Geometry check sheet. Reference: the model listing, model coordinates, mm. A direction names the side the tool comes from. Round coordinates to 2 decimals unless told otherwise and drop trailing zeros. Order: outer loops, then holes, each group sorted by start corner. A loop starts at its lowest first (then second) coordinate and runs counter-clockwise, first axis right, second up.
(1) Cross-section at A-A on x = 16. Enter the section's corners in (y, z), and give its area (3 significant figures).
(2) Cross-section at D-D on x = -41. Enter the section's corners in (y, z).
(3) Cross-section at C-C on y = 22.5. Enter the section's corners in (x, z), and give its area (3 significant figures).
(4) Set-up check for faces 5 (the face through (-1, 27.5, 1)), 6 (the face through (12.75, 14, 1)): record each of +Z, -Z, +X, -X, +Y, -Y from which the full face is reachable in a straight line by a thin tool's end or side.
(5) Cross-section at B-B on y = 0. Enter the section's corners in (x, z), and give its area (3 significant figures).
(6) Thickness scan on L1, parallel to X at y = 12, z = 2.9; L2, parallel to Y at x = -4.5, z = 2.55; L3, parallel to Y at x = 41, z = 2.3. Record the ranges inside material, lowest first.
(7) Draft check along X on faces 1 (the face through (-35.391, 16.796, 1.479)), 2 (the face through (1, 21, 1)), 3 (the face through (46, 0, 1)), 4 (the face through (-1, 0, 3)). Enter one of: pulls with the +X half, pulls with the -X half, needs draft (parallel to the pull), parting line crosses it, or undercut.
from build123d import *

# Parameters (mm, degrees)
SKETCH1_W           = 92
SKETCH1_H           = 55
SKETCH1_R           = 2
SKETCH1_R_2         = 1.5
BOSS_EXTRUDE1_DEPTH = 3


with BuildPart() as part:
    # Sketch1 → Boss-Extrude1 (new body)
    with BuildSketch(Plane.XY):
        Rectangle(SKETCH1_W, SKETCH1_H)
        with Locations((-34, 0)):
            Circle(SKETCH1_R, mode=Mode.SUBTRACT)
        with Locations((-14, 0)):
            Circle(SKETCH1_R, mode=Mode.SUBTRACT)
        with Locations((16, 0)):
            Circle(SKETCH1_R, mode=Mode.SUBTRACT)
        with Locations((-41, 22.5)):
            Circle(SKETCH1_R_2, mode=Mode.SUBTRACT)
        with Locations((41, 22.5)):
            Circle(SKETCH1_R_2, mode=Mode.SUBTRACT)
        with Locations((41, -22.5)):
            Circle(SKETCH1_R_2, mode=Mode.SUBTRACT)
        with Locations((-41, -22.5)):
            Circle(SKETCH1_R_2, mode=Mode.SUBTRACT)
        with BuildLine():
            Line((12.75, -21), (12.75, -6.199798384))
            ThreePointArc((12.75, -6.199798384), (11.050252532, -4.949747468), (9.800201616, -3.25))
            Line((9.800201616, -3.25), (-7.800201616, -3.25))
            ThreePointArc((-7.800201616, -3.25), (-9.050252532, -4.949747468), (-10.75, -6.199798384))
            Line((-10.75, -6.199798384), (-10.75, -21))
            Line((-10.75, -21), (12.75, -21))
        make_face(mode=Mode.SUBTRACT)
        with BuildLine():
            Line((-39.5, 4.330127019), (-39.5, 14.641883177))
            ThreePointArc((-39.5, 14.641883177), (-35.343145751, 16.843145751), (-33.141883177, 21))
            Line((-33.141883177, 21), (-17.25, 21))
            Line((-17.25, 21), (-17.25, 6.199798384))
            ThreePointArc((-17.25, 6.199798384), (-18.949747468, 4.949747468), (-20.199798384, 3.25))
            Line((-20.199798384, 3.25), (-27.800201616, 3.25))
            ThreePointArc((-27.800201616, 3.25), (-33.356495502, 6.970358812), (-39.5, 4.330127019))
        make_face(mode=Mode.SUBTRACT)
        with BuildLine():
            Line((-27.800201616, -3.25), (-20.199798384, -3.25))
            ThreePointArc((-20.199798384, -3.25), (-18.949747468, -4.949747468), (-17.25, -6.199798384))
            Line((-17.25, -6.199798384), (-17.25, -21))
            Line((-17.25, -21), (-33.141883177, -21))
            ThreePointArc((-33.141883177, -21), (-35.343145751, -16.843145751), (-39.5, -14.641883177))
            Line((-39.5, -14.641883177), (-39.5, -4.330127019))
            ThreePointArc((-39.5, -4.330127019), (-33.356495502, -6.970358812), (-27.800201616, -3.25))
        make_face(mode=Mode.SUBTRACT)
        with BuildLine():
            Line((19.25, -21), (19.25, -6.199798384))
            ThreePointArc((19.25, -6.199798384), (20.949747468, -4.949747468), (22.199798384, -3.25))
            Line((22.199798384, -3.25), (39.5, -3.25))
            Line((39.5, -3.25), (39.5, -14.641883177))
            ThreePointArc((39.5, -14.641883177), (35.343145751, -16.843145751), (33.141883177, -21))
            Line((33.141883177, -21), (19.25, -21))
        make_face(mode=Mode.SUBTRACT)
        with BuildLine():
            Line((39.5, 3.25), (39.5, 14.641883177))
            ThreePointArc((39.5, 14.641883177), (35.343145751, 16.843145751), (33.141883177, 21))
            Line((33.141883177, 21), (19.25, 21))
            Line((19.25, 21), (19.25, 6.199798384))
            ThreePointArc((19.25, 6.199798384), (20.949747468, 4.949747468), (22.199798384, 3.25))
            Line((22.199798384, 3.25), (39.5, 3.25))
        make_face(mode=Mode.SUBTRACT)
        with BuildLine():
            Line((-10.75, 21), (12.75, 21))
            Line((12.75, 21), (12.75, 6.199798384))
            ThreePointArc((12.75, 6.199798384), (11.050252532, 4.949747468), (9.800201616, 3.25))
            Line((9.800201616, 3.25), (-7.800201616, 3.25))
            ThreePointArc((-7.800201616, 3.25), (-9.050252532, 4.949747468), (-10.75, 6.199798384))
            Line((-10.75, 6.199798384), (-10.75, 21))
        make_face(mode=Mode.SUBTRACT)
    extrude(amount=BOSS_EXTRUDE1_DEPTH)


solid = part.part
Found:
1. outline: (-27.5, 0) - (-2, 0) - (-2, 3) - (-27.5, 3) - close; (2, 0) - (27.5, 0) - (27.5, 3) - (2, 3) - close
1. area: 153 mm2
2. outline: (-27.5, 0) - (-24, 0) - (-24, 3) - (-27.5, 3) - close; (-21, 0) - (21, 0) - (21, 3) - (-21, 3) - close; (24, 0) - (27.5, 0) - (27.5, 3) - (24, 3) - close
3. outline: (-46, 0) - (-42.5, 0) - (-42.5, 3) - (-46, 3) - close; (-39.5, 0) - (39.5, 0) - (39.5, 3) - (-39.5, 3) - close; (42.5, 0) - (46, 0) - (46, 3) - (42.5, 3) - close
3. area: 258 mm2
4. face 5: +Z, -Z, +X, -X, +Y
4. face 6: +Z, -Z
5. outline: (-46, 0) - (-36, 0) - (-36, 3) - (-46, 3) - close; (-32, 0) - (-16, 0) - (-16, 3) - (-32, 3) - close; (-12, 0) - (14, 0) - (14, 3) - (-12, 3) - close; (18, 0) - (46, 0) - (46, 3) - (18, 3) - close
5. area: 240 mm2
6. L1: x = -46 to -39.5, -17.25 to -10.75, 12.75 to 19.25, 39.5 to 46
6. L2: y = -27.5 to -21, -3.25 to 3.25, 21 to 27.5
6. L3: y = -27.5 to -24, -21 to 21, 24 to 27.5
7. face 1: undercut
7. face 2: undercut
7. face 3: pulls with the +X half
7. face 4: needs draft
